Check sheet for the modelled part. Datum: model origin and axes. Units: mm. Coordinates: 2 decimals unless noted, no trailing zeros. Write each loop counter-clockwise with the first axis right and the second up, starting at its lowest first coordinate (ties: lowest second). Pieces come first, ordered by that corner, then holes. Notation, with made-up numbers: (-34, -1.75) -> (-27, -1.75) arc R23 ccw to (-27, 11.25) -> close; hole circle Ø4 at (-36.75, -17). An arc over 180 degrees is marked (long way). One line per item, written item: value. Start each with the question number.
1) Sectioned sample at C-C on x = 78. Enter the section's corners in (y, z), plus the area to 3 significant figures.
2) Gauge pin test, flat end, axial feed: P1, Ø2, axis at x = -90.5, y = 1.5, coming from the +Z side (3 decimals). Record the tip position at first contact, or that the pin passes through.
3) Sectioned sample at B-B on y = 1.8. Give the number of separate pieces and of enclosed holes in the cut face, plus the area to 3 significant figures.
4) Sectioned sample at D-D on z = -64. Enter the section's corners in (x, y).
5) Scan lines: line 1 along X through (y, z) = (2, -121); line 2 along Z through (x, y) = (55, 3.55); line 3 along X through (y, z) = (4.2, 7). Record each from-to range of solid material in increasing order. Write a range as [from, to].
6) Sectioned sample at A-A on z = 3.5. Enter the section's corners in (x, y), plus the area to 3 significant figures.
```python
from build123d import *

# Parameters (mm, degrees)
SKETCH_2_R          = 2.25
EXTRUDE_2_DEPTH     = 5
SKETCH_3_W          = 15
SKETCH_3_H          = 100
CUT_EXTRUDE_1_DEPTH = 5
CUT_EXTRUDE_2_DEPTH = 5


with BuildPart() as part:
    # 草圖2 → 填料-伸長2 (new body)
    with BuildSketch(Plane(origin=(0, 0, 0), x_dir=(1, 0, 0), z_dir=(0, 1, 0))):
        Polygon((-150, 150), (150, 150), (150, -50), (70, -150), (-70, -150), (-150, -50), align=None)
        with Locations((-105, 121)):
            Circle(SKETCH_2_R, mode=Mode.SUBTRACT)
        with Locations((-105, 79)):
            Circle(SKETCH_2_R, mode=Mode.SUBTRACT)
        with Locations((-55, 79)):
            Circle(SKETCH_2_R, mode=Mode.SUBTRACT)
        with Locations((-55, 121)):
            Circle(SKETCH_2_R, mode=Mode.SUBTRACT)
        with Locations((55, 121)):
            Circle(SKETCH_2_R, mode=Mode.SUBTRACT)
        with Locations((55, 79)):
            Circle(SKETCH_2_R, mode=Mode.SUBTRACT)
        with Locations((105, 121)):
            Circle(SKETCH_2_R, mode=Mode.SUBTRACT)
        with Locations((105, 79)):
            Circle(SKETCH_2_R, mode=Mode.SUBTRACT)
    extrude(amount=EXTRUDE_2_DEPTH)

    # 草圖3 → 除料-伸長1 (cut)
    with BuildSketch(Plane(origin=(0, 5, 0), x_dir=(1, 0, 0), z_dir=(0, 1, 0))):
        with Locations((-142.5, 100)):
            Rectangle(SKETCH_3_W, SKETCH_3_H)
        with Locations((142.5, 100)):
            Rectangle(SKETCH_3_W, SKETCH_3_H)
    extrude(amount=-CUT_EXTRUDE_1_DEPTH, mode=Mode.SUBTRACT)

    # 草圖4 → 除料-伸長2 (cut)
    with BuildSketch(Plane(origin=(0, 5, 0), x_dir=(1, 0, 0), z_dir=(0, 1, 0))):
        with BuildLine():
            Line((-95.5, 45), (-95.5, -15))
            ThreePointArc((-95.5, -15), (-97.5, -17), (-99.5, -15))
            Line((-99.5, -15), (-99.5, 45))
            ThreePointArc((-99.5, 45), (-97.5, 47), (-95.5, 45))
        make_face()
        with BuildLine():
            Line((-64.5, 45), (-64.5, -15))
            ThreePointArc((-64.5, -15), (-62.5, -17), (-60.5, -15))
            Line((-60.5, -15), (-60.5, 45))
            ThreePointArc((-60.5, 45), (-62.5, 47), (-64.5, 45))
        make_face()
        with BuildLine():
            Line((95.5, 45), (95.5, -15))
            ThreePointArc((95.5, -15), (97.5, -17), (99.5, -15))
            Line((99.5, -15), (99.5, 45))
            ThreePointArc((99.5, 45), (97.5, 47), (95.5, 45))
        make_face()
        with BuildLine():
            Line((64.5, 45), (64.5, -15))
            ThreePointArc((64.5, -15), (62.5, -17), (60.5, -15))
            Line((60.5, -15), (60.5, 45))
            ThreePointArc((60.5, 45), (62.5, 47), (64.5, 45))
        make_face()
    extrude(amount=-CUT_EXTRUDE_2_DEPTH, mode=Mode.SUBTRACT)


solid = part.part
```
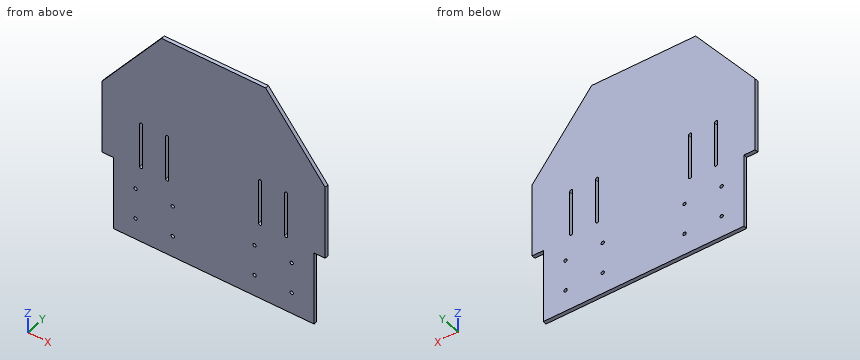
Answers:
1. outline: (0, -150) -> (5, -150) -> (5, 140) -> (0, 140) -> close
1. area: 1,450 mm2
2. P1: stops at z = 125.625
3. separate pieces: 1
3. enclosed holes: 12
3. area: 77,900 mm2
4. outline: (-135, 0) -> (135, 0) -> (135, 5) -> (-135, 5) -> close
5. line 1: x = [-135, -107.25], [-102.75, -57.25], [-52.75, 52.75], [57.25, 102.75], [107.25, 135]
5. line 2: z = [-150, -123.25], [-118.75, -81.25], [-76.75, 150]
5. line 3: x = [-150, -99.5], [-95.5, -64.5], [-60.5, 60.5], [64.5, 95.5], [99.5, 150]
6. outline: (-150, 0) -> (-99.5, 0) -> (-99.5, 5) -> (-150, 5) -> close; (-95.5, 0) -> (-64.5, 0) -> (-64.5, 5) -> (-95.5, 5) -> close; (-60.5, 0) -> (60.5, 0) -> (60.5, 5) -> (-60.5, 5) -> close; (64.5, 0) -> (95.5, 0) -> (95.5, 5) -> (64.5, 5) -> close; (99.5, 0) -> (150, 0) -> (150, 5) -> (99.5, 5) -> close
6. area: 1,420 mm2
